from build123d import *

# Parameters (mm, degrees)
CROQUIS1_R              = 25
SALIENTE_EXTRUIR1_DEPTH = 2.8
CROQUIS2_W              = 2.75
CROQUIS2_H              = 18
CORTAR_EXTRUIR1_DEPTH   = 3.8
MATRIZC1_COUNT          = 8


with BuildPart() as part:
    # Croquis1 → Saliente-Extruir1 (new body)
    with BuildSketch(Plane.XY):
        Circle(CROQUIS1_R)
    extrude(amount=SALIENTE_EXTRUIR1_DEPTH)

    # Croquis2 → Cortar-Extruir1 (cut, through all)
    with BuildSketch(Plane.XY):
        with Locations((0, 25)):
            Rectangle(CROQUIS2_W, CROQUIS2_H)
    cortar_extruir1 = extrude(amount=CORTAR_EXTRUIR1_DEPTH, mode=Mode.SUBTRACT)

    # MatrizC1: Cortar-Extruir1 ×8 about axis
    matrizc1_axis = Axis((0, 0, 0), (0, 0, 1))
    for i in range(1, MATRIZC1_COUNT):
        add(cortar_extruir1.rotate(matrizc1_axis, i * 360 / MATRIZC1_COUNT), mode=Mode.SUBTRACT)


solid = part.part
For this review, take the finished solid that the model builds, in its own axes (mm). A direction names the side the tool comes from. Round coordinates to 2 decimals unless told otherwise and drop trailing zeros. Write each loop counter-clockwise with the first axis right and the second up, starting at its lowest first coordinate (ties: lowest second). Pieces come first, ordered by that corner, then holes. Notation, with made-up numbers: (34, 50) -> (44, 50) arc R15 cw to (44, 62) -> close; hole circle Ø11 at (18.5, 4.5). An arc over 180 degrees is marked (long way). Use CSV: the item, a comma, the result in double quotes.
(1) Clearance check with flat-ended pins moving along their axes: P1, Ø1.4, axis at y = -22.5, z = 1.5, coming from the -X side; P2, Ø10, axis at x = 12.5, y = -13, coming from the +Z side; P3, Ø1.4, axis at y = 0.5, z = 1, coming from the -X side; P4, Ø0.8, axis at x = 0.5, z = 0.5, coming from the +Y side. State where each tip first meets the part, or that it passes through.
Computed values:
P1,"x = -12.24"
P2,"z = 2.8"
P3,"x = -16"
P4,"y = 16"
(2) Consider section B-B, the plane y = 18. Give the boundary of the cut face in (x, z) (3 decimals).
Computed values:
outline,"(-16.055, 0) -> (-1.375, 0) -> (-1.375, 2.8) -> (-16.055, 2.8) -> close; (1.375, 0) -> (16.055, 0) -> (16.055, 2.8) -> (1.375, 2.8) -> close"
(3) Draft analysis for pull direction Y (two halves, no side actions). For faces 4 (the face through (9.68, 23.05, 1.38)), 5 (the face through (1.375, -20, 1)), 6 (the face through (16, 0, 1)), 7 (the face through (-23.14, -9.46, 1.38)), state which applies: +Y half, -Y half, draft (parallel to the pull), parting line (faces both ways), or undercut.
Computed values:
face 4,"+Y half"
face 5,"draft"
face 6,"undercut"
face 7,"-Y half"
(4) Consider section C-C, the plane x = -20.5. Give the boundary of the cut face in (y, z) (3 decimals), plus the area to 3 significant figures.
Computed values:
outline,"(-14.309, 0) -> (-1.375, 0) -> (-1.375, 2.8) -> (-14.309, 2.8) -> close; (1.375, 0) -> (14.309, 0) -> (14.309, 2.8) -> (1.375, 2.8) -> close"
area,"72.4 mm²"
(5) To check wall thickness, follow L1, parallel to Y at x = 13, z = 1.5; L2, parallel to Y at x = 15, z = 2.2; L3, parallel to X at y = -11, z = 1.6. State the ranges of each line that lie inside material, in increasing order. Write a range as [from, to].
Computed values:
L1,"[-21.35, -14.94], [-11.06, 11.06], [14.94, 21.35]"
L2,"[-20, -16.94], [-13.06, 13.06], [16.94, 20]"
L3,"[-22.45, -12.94], [-11.63, 11.63], [12.94, 22.45]"
(6) Consider section A-A, the plane y = -15. Give the boundary of the cut face in (x, z).
Computed values:
outline,"(-20, 0) -> (-16.94, 0) -> (-16.94, 2.8) -> (-20, 2.8) -> close; (-13.06, 0) -> (13.06, 0) -> (13.06, 2.8) -> (-13.06, 2.8) -> close; (16.94, 0) -> (20, 0) -> (20, 2.8) -> (16.94, 2.8) -> close"
(7) For faces 1 (the face through (20, 1.375, 1)), 2 (the face through (-13.466, 15.41, 1.38)), 3 (the face through (1.375, 20, 1)), list the 3-axis set-ups (+Z, -Z, +X, -X, +Y, -Y) from which the entire face can be reached by the end or side of a thin tool; tool diameter is ignored.
Computed values:
face 1,"+Z, -Z, +X"
face 2,"+Z, -Z"
face 3,"+Z, -Z, +Y"
